Model file for the job. Use its own axes, mm. A direction names the side the tool comes from. Give positions to 0.01 mm unless a question says otherwise; leave off trailing zeros. Loops run counter-clockwise (first coordinate to the right, second up) from the corner with the lowest first, then second, coordinate; pieces in that order, holes last. Notation, with made-up numbers: M 30.25,37 L 67.25,37 A25 ccw 67.25,58 Z; hole C 42.5,-10.75 d5. An arc over 180 degrees is marked long. Answer in a Markdown table with one row per item.
```python
from build123d import *

# Parameters (mm, degrees)
BASE_FLANGE1_DEPTH = 20.1168
SKETCH6_R          = 2.4892
CUT_EXTRUDE1_DEPTH = 66.121602646
SKETCH7_R          = 5.08
CUT_EXTRUDE2_DEPTH = 65.599391106
FILLET1_R          = 3.175


# Read off the part's stored shape, not the designer's step: Base-Flange1
with BuildPart() as part:
    # Base-Flange1 outline → Base-Flange1 (new body)
    with BuildSketch(Plane(origin=(0, 0, 0), x_dir=(1, 0, 0), z_dir=(0, 1, 0))):
        with BuildLine():
            Line((3.429, 0), (50.8, 0))
            Line((50.8, 0), (50.8, 2.667))
            Line((50.8, 2.667), (3.429, 2.667))
            ThreePointArc((3.429, 2.667), (2.890184633, 2.890184633), (2.667, 3.429))
            Line((2.667, 3.429), (2.667, 38.1))
            Line((2.667, 38.1), (0, 38.1))
            Line((0, 38.1), (0, 3.429))
            ThreePointArc((0, 3.429), (1.004330847, 1.004330847), (3.429, 0))
        make_face()
    extrude(amount=BASE_FLANGE1_DEPTH)

    # Sketch6 → Cut-Extrude1 (cut, through all)
    with BuildSketch(Plane(origin=(0, 0, -2.667), x_dir=(-1, 0, 0), z_dir=(0, 0, -1))):
        with Locations((-38.1, 10.0584)):
            Circle(SKETCH6_R)
        with Locations((-25.4, 10.0584)):
            Circle(SKETCH6_R)
        with Locations((-12.7, 10.0584)):
            Circle(SKETCH6_R)
    extrude(amount=-CUT_EXTRUDE1_DEPTH, mode=Mode.SUBTRACT)

    # Sketch7 → Cut-Extrude2 (cut, through all)
    with BuildSketch(Plane(origin=(2.667, 0, 0), x_dir=(0, 0, -1), z_dir=(1, 0, 0))):
        with Locations((25.4, 10.0584)):
            Circle(SKETCH7_R)
    extrude(amount=-CUT_EXTRUDE2_DEPTH, mode=Mode.SUBTRACT)

    # Fillet1
    fillet1_edges = [part.edges().sort_by_distance(p)[0] for p in [
        (1.3335, 20.1168, -38.1),
        (1.3335, 0, -38.1),
        (50.8, 20.1168, -1.3335),
        (50.8, 0, -1.3335),
    ]]
    fillet(fillet1_edges, radius=FILLET1_R)


solid = part.part
```
(1) Saw through at A-A, the plane x = 38.1. Give the cut face in (y, z).
Established:
| item | result |
|---|---|
| outline | M 0,-2.67 L 7.57,-2.67 L 7.57,0 L 0,0 Z; M 12.55,-2.67 L 20.12,-2.67 L 20.12,0 L 12.55,0 Z |
(2) Saw through at C-C, the plane y = 6. Give the cut face in (x, z), and give its area (3 significant figures).
Established:
| item | result |
|---|---|
| outline | M 0,-38.1 L 2.67,-38.1 L 2.67,-28.46 L 0,-28.46 Z; M 0,-22.34 L 2.67,-22.34 L 2.67,-3.43 A0.76 cw 3.43,-2.67 L 50.8,-2.67 L 50.8,0 L 3.43,0 A3.43 ccw 0,-3.43 Z |
| area | 211 mm2 |
(3) Saw through at B-B, the plane z = -25.4. Give the cut face in (x, y), and give its area (3 significant figures).
Established:
| item | result |
|---|---|
| outline | M 0,0 L 2.67,0 L 2.67,4.98 L 0,4.98 Z; M 0,15.14 L 2.67,15.14 L 2.67,20.12 L 0,20.12 Z |
| area | 26.6 mm2 |
(4) Flat gauge pins, fed straight in: P1, Ø5.5, axis at x = 38.1, y = 10.06, coming from the -Z side; P2, Ø10, axis at y = 6.5, z = -24, coming from the +X side. Where does each tip first touch, or does it go through?
Established:
| item | result |
|---|---|
| P1 | stops at z = -2.67 |
| P2 | stops at x = 2.67 |
(5) Wall check: L1, parallel to Y at x = 0.95, z = -25.4; L2, parallel to X at y = 14.5, z = -14; L3, parallel to Z at x = 45.5, y = 17.25. Give the ranges that are in metal, low to high.
Established:
| item | result |
|---|---|
| L1 | y = 0 to 4.98, 15.14 to 20.12 |
| L2 | x = 0 to 2.67 |
| L3 | z = -2.67 to 0 |
(6) Which spindle directions (+Z, -Z, +X, -X, +Y, -Y) get a long thin tool onto all of the face, cutting with end or side? Do faces 4 (the cylindrical face through (1.315, 19.211, -37.145)), 5 (the flat face through (2.667, 12.2, -20.5)). Say none if no direction does.
Established:
| item | result |
|---|---|
| face 4 | -Z, +X, -X, +Y |
| face 5 | -Z, +X, +Y, -Y |
(7) Mould opens along X. For faces 1 (the cylindrical face through (49.85, 0.91, -1.35)), 2 (the flat face through (27.4, 7.7, -2.667)), 3 (the cylindrical face through (13.24, 7.63, -1.35)) say: pulls with the +X half, pulls with the -X half, needs draft (parallel to the pull), parting line crosses it, or undercut.
Established:
| item | result |
|---|---|
| face 1 | pulls with the +X half |
| face 2 | needs draft |
| face 3 | undercut |
(8) Saw through at D-D, the plane y = 9. Give the cut face in (x, z).
Established:
| item | result |
|---|---|
| outline | M 0,-38.1 L 2.67,-38.1 L 2.67,-30.37 L 0,-30.37 Z; M 0,-20.43 L 2.67,-20.43 L 2.67,-3.43 A0.76 cw 3.43,-2.67 L 10.45,-2.67 L 10.45,0 L 3.43,0 A3.43 ccw 0,-3.43 Z; M 14.95,-2.67 L 23.15,-2.67 L 23.15,0 L 14.95,0 Z; M 27.65,-2.67 L 35.85,-2.67 L 35.85,0 L 27.65,0 Z; M 40.35,-2.67 L 50.8,-2.67 L 50.8,0 L 40.35,0 Z |
